Autodesk Inventor part; units mm, degrees
ref_plane "Work Plane1" through (0, 0, 3.175) normal (0, 0, -1) x (-1, 0, 0)
ref_plane "Work Plane2" through (0, 0, 7.9375) normal (0, 0, -1) x (-1, 0, 0)
ref_plane "YZ Plane" through (0, 0, 0) normal (1, 0, 0) x (0, 1, 0)
sketch "Sketch1" plane through (0, 0, 0) normal (0, 0, 1) x (1, 0, 0)
  circle A0 centre (0, 0) radius 3.3655
  circle A1 centre (0, 0) radius 1.905
  circle A2 centre (-15.875, 0) radius 1.905
  line L0 (-15.875, -3.8861) -> (-19.2405, -1.9431)
  line L1 (-19.2405, -1.9431) -> (-19.2405, 1.9431)
  line L2 (-19.2405, 1.9431) -> (-15.875, 3.8861)
  line L3 (-15.875, 3.8861) -> (-12.5095, 1.9431)
  line L4 (-12.5095, 1.9431) -> (-12.5095, -1.9431)
  line L5 (-12.5095, -1.9431) -> (-15.875, -3.8861)
  line L6 (-22.86, 5.715) -> (6.985, 5.715)
  line L7 (6.985, 5.715) -> (6.985, -4.445)
  line L8 (6.985, -4.445) -> (-22.86, -4.445)
  line L9 (-22.86, -4.445) -> (-22.86, 5.715)
  dimension "d0" = 6.731
  dimension "d1" = 3.81
  dimension "d2" = 3.81
  dimension "d3" = 6.731
  dimension "d4" = 15.875
  dimension "d5" = 10.16
  dimension "d6" = 29.845
  dimension "d30" = 4.445
  dimension "d31" = 6.985
extrude "Extrusion1" add sketch "Sketch1" along normal blind 15.875 contours L6 L7 L8 L9
ref_plane "Work Plane1" through (0, 0, 3.175) normal (0, 0, -1) x (-1, 0, 0)
sketch "Sketch2" plane through (0, 0, 3.175) normal (0, 0, -1) x (-1, 0, 0)
  circle A0 centre (0, 0) radius 1.905
  circle A1 centre (0, 0) radius 3.3655
  circle A2 centre (15.875, 0) radius 1.905
  line L0 (19.2405, 1.9431) -> (19.2405, -1.9431)
  line L1 (19.2405, -1.9431) -> (15.875, -3.8861)
  line L2 (15.875, -3.8861) -> (12.5095, -1.9431)
  line L3 (12.5095, -1.9431) -> (12.5095, 1.9431)
  line L4 (12.5095, 1.9431) -> (15.875, 3.8861)
  line L5 (15.875, 3.8861) -> (19.2405, 1.9431)
  circle A3 centre (0, 0) radius 3.3655
  line L6 (22.86, 5.715) -> (-6.985, 5.715)
  line L7 (-6.985, 5.715) -> (-6.985, -4.445)
  line L8 (-6.985, -4.445) -> (22.86, -4.445)
  line L9 (22.86, -4.445) -> (22.86, 5.715)
extrude "Extrusion2" add sketch "Sketch2" against normal blind 9.525 contours A1 | L0 L1 L2 L3 L4 L5
ref_plane "Work Plane2" through (0, 0, 7.9375) normal (0, 0, -1) x (-1, 0, 0)
sketch "Sketch4" plane through (0, 0, 7.9375) normal (0, 0, -1) x (-1, 0, 0)
  circle A0 centre (0, 0) radius 1.905 construction
  circle A1 centre (15.875, 0) radius 1.905 construction
  line L0 (-6.985, -4.445) -> (-6.985, 5.715) construction
  line L1 (-6.985, 5.715) -> (22.86, 5.715) construction
  line L2 (22.86, 5.715) -> (22.86, -4.445) construction
  line L3 (22.86, -4.445) -> (-6.985, -4.445) construction
  line L4 (22.86, 5.715) -> (-6.985, 5.715)
  line L5 (-6.985, -4.445) -> (22.86, -4.445)
  arc A2 (10.795, 5.715) -> (14.351, -4.445) centre (26.0305, 5.3451) ccw
  line L6 (10.795, 5.715) -> (3.81, 5.715)
  line L7 (3.81, 5.715) -> (3.81, -4.445)
  line L8 (3.81, -4.445) -> (14.351, -4.445)
  dimension "d14" = 15.24
  dimension "d15" = 12.065
  dimension "d16" = 8.509
  dimension "d17" = 10.795
extrude "Extrusion3" cut sketch "Sketch4" along normal mid plane 4.445
fillet "Fillet4" radius 1.27 4 edges at (-7.3025, 5.715, 5.715) (-7.3025, 5.715, 10.16) (-3.81, 5.715, 7.9375) (-10.795, 5.715, 7.9375)
chamfer "Chamfer1" distance 4.826 distance2 2.794 1 edges at (-22.86, 5.715, 7.9375) measured on face at (-19.2698, 5.715, 6.7733)
chamfer "Chamfer2" distance 4.826 distance2 2.794 1 edges at (6.985, 5.715, 7.9375) measured on face at (3.81, 5.715, 9.1017)
fillet "Fillet5" radius 1.27 4 edges at (-18.034, 5.715, 7.9375) (-22.86, 2.921, 7.9375) (2.159, 5.715, 7.9375) (6.985, 2.921, 7.9375)
fillet "Fillet6" radius 0.635 18 edges at (-18.0223, 5.6715, 15.875) (-20.2778, 4.416, 15.875) (-22.6902, 2.8231, 15.875) (-22.86, -1.1281, 15.875) (2.1473, 5.6715, 15.875) (4.4028, 4.416, 15.875) (6.8152, 2.8231, 15.875) (6.985, -1.1281, 15.875) (-7.9375, 5.715, 15.875) (2.1473, 5.6715, 0) (4.4028, 4.416, 0) (6.8152, 2.8231, 0) (6.985, -1.1281, 0) (-18.0223, 5.6715, 0) (-20.2778, 4.416, 0) (-22.6902, 2.8231, 0) (-22.86, -1.1281, 0) (-7.9375, 5.715, 0)
sketch "Sketch5" plane through (0, 0, 0) normal (0, 0, -1) x (-1, 0, 0)
  line L0 (5.715, 5.715) -> (10.16, 5.715)
  line L1 (10.16, 5.715) -> (10.16, 3.429)
  line L2 (10.16, 3.429) -> (5.715, 3.429)
  line L3 (5.715, 3.429) -> (5.715, 5.715)
  circle A0 centre (15.875, 0) radius 1.905 construction
  circle A1 centre (0, 0) radius 1.905 construction
  line L4 (0, 0) -> (15.875, 0) construction
  line L5 (17.6929, 5.715) -> (-1.8179, 5.715) construction
  point P0 (7.9375, 3.429)
  point P1 (7.9375, 0)
  dimension "d32" = 4.445
  dimension "d33" = 2.286
extrude "Extrusion4" cut sketch "Sketch5" against normal up to surface (5.715 mm away)
fillet "Fillet7" radius 0.635 10 edges at (-5.715, 5.529, 0.186) (-5.715, 5.715, 2.54) (-5.715, 5.343, 5.343) (-5.715, 3.937, 5.715) (-5.715, 4.2545, 0) (-10.16, 5.529, 0.186) (-10.16, 5.715, 2.54) (-10.16, 5.343, 5.343) (-10.16, 3.937, 5.715) (-10.16, 4.2545, 0)
fillet "Fillet8" radius 1.27 1 edges at (-7.9375, 3.429, 5.715)
properties part number "CarriageImproved" material "ABS Plastic"
Geometry: final body of the model. Coordinates: model frame, mm. A direction names the side the tool comes from. Give positions to 0.01 mm unless a question says otherwise; leave off trailing zeros. Order: outer loops, then holes, each group sorted by start corner. A loop starts at its lowest first (then second) coordinate and runs counter-clockwise, first axis right, second up. Notation, with made-up numbers: M 25.25,88 L 49.25,88 A28 ccw 49.25,123 Z; hole C 3,4 d1. An arc over 180 degrees is marked long. Answer as CSV lines item,"result". Start each with the question number.
1) Mould query, pull axis Y, two halves, no side actions, for faces 4 (the flat face through (-3.81, 0, 8)), 5 (the flat face through (-8, 3.429, 2)), 6 (the flat face through (-17.58, 2.9, 1.57)). Classes: +Y half, -Y half, draft (parallel to the pull), parting line (faces both ways), or undercut.
2) Cut plane A-A (z = 9). Output: boundary loops of the cut face in (x, y) (3 decimals), then the cut area to 3 significant figures.
3) Line query: line 1 (X direction, y = 0, z = 14.65) (1 decimal); line 2 (Z direction, x = -7, y = -2) (3 decimals); line 3 (Y direction, x = 0, z = 0.95) (1 decimal). Output: solid intervals per line, ascending. Write a range as from..to.
4) Set-up query: faces 1 (the flat face through (-19.24, 0, 2)), 2 (the flat face through (0, -2.2, 12.7)), 3 (the cylindrical face through (0.41, -1.86, 7.87)). Return all of +Z, -Z, +X, -X, +Y, -Y with unobstructed straight access to the full face (end or side cutting, diameter ignored); none if empty.
5) Cut plane C-C (x = -4.5). Output: boundary loops of the cut face in (y, z) (3 decimals), then the cut area to 3 significant figures.
6) First-contact query: P1, Ø2, axis at x = -16.5, y = -0.5, coming from the -Z side; P2, Ø5.5, axis at x = 0, y = 0, coming from the -Z side (3 decimals); P3, Ø1.5, axis at y = 4.5, z = 2, coming from the -X side; P4, Ø2, axis at x = -8.5, z = 2, coming from the +Y side. Flat tips, straight axial feed; report the tip coordinate or a pass-through.
7) Cut plane D-D (y = 1.5). State how many separate pieces and enclosed holes the cut face has, then the cut area to 3 significant figures.
8) Cut plane B-B (x = 0). Output: boundary loops of the cut face in (y, z) (1 decimal).
Findings below:
1,face 4,"draft"
1,face 5,"+Y half"
1,face 6,"undercut"
2,outline,"M -22.86,-4.445 L -14.351,-4.445 A15.24 ccw -10.822,4.363 A1.27 ccw -12.09,5.715 L -17.693,5.715 A1.27 ccw -18.329,5.544 L -22.226,3.288 A1.27 ccw -22.86,2.189 Z; M -3.81,-4.445 L 6.985,-4.445 L 6.985,2.189 A1.27 ccw 6.351,3.288 L 2.454,5.544 A1.27 ccw 1.818,5.715 L -2.54,5.715 A1.27 ccw -3.81,4.445 Z; hole C -15.875,0 d3.81; hole C 0,0 d3.81"
2,area,"184 mm²"
3,line 1,"x = -22.9..-19.2, -12.5..-3.4, 3.4..7"
3,line 2,"z = 0..5.715, 10.16..15.875"
3,line 3,"y = -4.4..-3.4, 3.4..5.7"
4,face 1,"-Z"
4,face 2,"+Z"
4,face 3,"+Z, -Z"
5,outline,"M -4.445,0 L 5.08,0 A0.635 ccw 5.715,0.635 L 5.715,4.445 A1.27 ccw 4.445,5.715 L -4.445,5.715 Z; M -4.445,10.16 L 4.445,10.16 A1.27 ccw 5.715,11.43 L 5.715,15.24 A0.635 ccw 5.08,15.875 L -4.445,15.875 Z"
5,area,"115 mm²"
6,P1,"passes through"
6,P2,"stops at z = 3.175"
6,P3,"stops at x = -21.43"
6,P4,"stops at y = 3.43"
7,separate pieces,"3"
7,enclosed holes,"1"
7,area,"314 mm²"
8,outline,"M -4.4,0 L -3.4,0 L -3.4,3.2 L -1.9,3.2 L -1.9,12.7 L -3.4,12.7 L -3.4,15.9 L -4.4,15.9 Z; M 1.9,3.2 L 3.4,3.2 L 3.4,0 L 5.1,0 A0.6 ccw 5.7,0.6 L 5.7,15.2 A0.6 ccw 5.1,15.9 L 3.4,15.9 L 3.4,12.7 L 1.9,12.7 Z"
